Build history of the part. All positions in model axes, mm. A direction names the side the tool comes from. Give positions to 0.01 mm unless a question says otherwise; leave off trailing zeros. Write each loop counter-clockwise with the first axis right and the second up, starting at its lowest first coordinate (ties: lowest second). Pieces come first, ordered by that corner, then holes.
from build123d import *

# Parameters (mm, degrees)
SKETCH1_R                   = 25.4
BOSS_EXTRUDE1_DEPTH         = 152.4
SKETCH3_W                   = 25.4
SKETCH3_H                   = 88.9
CUT_EXTRUDE1_DEPTH          = 102.6
CUT_EXTRUDE1_DEPTH_BACK     = 102.6
F_1_4_0_25_DIAMETER_HOLE1_D = 6.35
SKETCH4_W                   = 25.4
SKETCH4_H                   = 101.6
CUT_EXTRUDE2_DEPTH          = 18.196861737


with BuildPart() as part:
    # Sketch1 → Boss-Extrude1 (new body)
    with BuildSketch(Plane.XY):
        with BuildLine():
            Line((-76.2, -38.1), (-76.2, -12.7))
            ThreePointArc((-76.2, -12.7), (-57.601280605, 32.201280605), (-12.7, 50.8))
            Line((-12.7, 50.8), (12.7, 50.8))
            ThreePointArc((12.7, 50.8), (57.601280605, 32.201280605), (76.2, -12.7))
            Line((76.2, -12.7), (76.2, -38.1))
            Line((76.2, -38.1), (101.6, -38.1))
            Line((101.6, -38.1), (101.6, -50.8))
            ThreePointArc((101.6, -50.8), (0, -55.296861637), (-101.6, -50.8))
            Line((-101.6, -50.8), (-101.6, -38.1))
            Line((-101.6, -38.1), (-76.2, -38.1))
        make_face()
        Circle(SKETCH1_R, mode=Mode.SUBTRACT)
    extrude(amount=BOSS_EXTRUDE1_DEPTH)

    # Sketch3 → Cut-Extrude1 (cut, two sides)
    with BuildSketch(Plane(origin=(0, 0, 0), x_dir=(0, 0, -1), z_dir=(1, 0, 0))) as cut_extrude1_sk:
        with Locations((-114.3, 6.35)):
            Rectangle(SKETCH3_W, SKETCH3_H)
        with Locations((-38.1, 6.35)):
            Rectangle(SKETCH3_W, SKETCH3_H)
    extrude(amount=CUT_EXTRUDE1_DEPTH, mode=Mode.SUBTRACT)
    extrude(cut_extrude1_sk.sketch, amount=-CUT_EXTRUDE1_DEPTH_BACK, mode=Mode.SUBTRACT)

    # 1/4 (0.25) Diameter Hole1 (through all)
    with Locations(Plane(origin=(0, -38.1, 0), x_dir=(1, 0, 0), z_dir=(0, 1, 0))):
        with Locations((-88.9, -12.7), (-88.9, -139.7), (88.9, -12.7), (88.9, -139.7)):
            Hole(F_1_4_0_25_DIAMETER_HOLE1_D / 2)

    # Sketch4 → Cut-Extrude2 (cut, through all)
    with BuildSketch(Plane(origin=(0, -38.1, 0), x_dir=(1, 0, 0), z_dir=(0, 1, 0))):
        with Locations((-88.9, -76.2)):
            Rectangle(SKETCH4_W, SKETCH4_H)
        with Locations((88.9, -76.2)):
            Rectangle(SKETCH4_W, SKETCH4_H)
    extrude(amount=-CUT_EXTRUDE2_DEPTH, mode=Mode.SUBTRACT)


solid = part.part
1. Drop flat-ended pins along their axis: pin 1 (20.5 mm diameter, centred on x = 94.5, z = 9.5, fed in from +Y); pin 2 (12.5 mm diameter, centred on y = -20, z = 146, fed in from -X); pin 3 (10 mm diameter, centred on y = 16.5, z = 70.5, fed in from -X). Give the stop position or say it passes through.
2. Mould opens along Z. For faces 5 (the face through (24, -13, 152.4)), 6 (the face through (-89, -45, 25.4)), 7 (the face through (76.2, -25, 13)) say: pulls with the +Z half, pulls with the -Z half, needs draft (parallel to the pull), parting line crosses it, or undercut.
3. Saw through at C-C on y = 0. Give the cut face in (x, z), plus the area to 3 significant figures.
4. 3-axis set-ups, long thin cutter, end or side, ignore diameter. For faces 1 (the face through (-89, -45, 127)), 2 (the face through (-76.2, -26, 13)), 3 (the face through (-1, -38.1, 38)), 4 (the face through (76.2, -25, 140)): which of +Z, -Z, +X, -X, +Y, -Y reach the whole face in a straight line?
5. Drill centre lines: line 1 along Z through (x, y) = (13, 29.5); line 2 along X through (y, z) = (-43.25, 139.7) (3 decimals); line 3 along Z through (x, y) = (-88.9, -41.5) (3 decimals). Where is each one in solid material? Low to high.
6. Saw through at D-D on z = 12.7. Give the cut face in (x, y) (3 decimals).
7. Saw through at B-B on x = 0. Give the cut face in (y, z), plus the area to 3 significant figures.
8. Saw through at A-A on z = 131. Give the cut face in (x, y), plus the area to 3 significant figures.
Outcome:
1. pin 1: stops at y = -38.1
1. pin 2: stops at x = -76.2
1. pin 3: stops at x = -71.41
2. face 5: pulls with the +Z half
2. face 6: undercut
2. face 7: needs draft
3. outline: (-74.92, 0) - (-25.4, 0) - (-25.4, 25.4) - (-74.92, 25.4) - close; (-74.92, 50.8) - (-25.4, 50.8) - (-25.4, 101.6) - (-74.92, 101.6) - close; (-74.92, 127) - (-25.4, 127) - (-25.4, 152.4) - (-74.92, 152.4) - close; (25.4, 0) - (74.92, 0) - (74.92, 25.4) - (25.4, 25.4) - close; (25.4, 50.8) - (74.92, 50.8) - (74.92, 101.6) - (25.4, 101.6) - close; (25.4, 127) - (74.92, 127) - (74.92, 152.4) - (25.4, 152.4) - close
3. area: 10,100 mm2
4. face 1: -X, +Y, -Y
4. face 2: +Z, -Z, -X, +Y
4. face 3: +X, -X, +Y
4. face 4: +Z, -Z, +X, +Y
5. line 1: z = 0 to 25.4, 50.8 to 101.6, 127 to 152.4
5. line 2: x = -101.6 to -92.075, -85.725 to 85.725, 92.075 to 101.6
5. line 3: z = 0 to 9.525, 15.875 to 25.4, 127 to 136.525, 142.875 to 152.4
6. outline: (-101.6, -50.8) arc R1150 ccw to (-92.075, -51.605) - (-92.075, -38.1) - (-101.6, -38.1) - close; (-85.725, -52.097) arc R1150 ccw to (85.725, -52.097) - (85.725, -38.1) - (76.2, -38.1) - (76.2, -12.7) arc R63.5 ccw to (12.7, 50.8) - (-12.7, 50.8) arc R63.5 ccw to (-76.2, -12.7) - (-76.2, -38.1) - (-85.725, -38.1) - close; (92.075, -51.605) arc R1150 ccw to (101.6, -50.8) - (101.6, -38.1) - (92.075, -38.1) - close; hole circle Ø50.8 at (0, 0)
7. outline: (-55.3, 0) - (-25.4, 0) - (-25.4, 25.4) - (-38.1, 25.4) - (-38.1, 50.8) - (-25.4, 50.8) - (-25.4, 101.6) - (-38.1, 101.6) - (-38.1, 127) - (-25.4, 127) - (-25.4, 152.4) - (-55.3, 152.4) - close; (25.4, 0) - (50.8, 0) - (50.8, 25.4) - (25.4, 25.4) - close; (25.4, 50.8) - (50.8, 50.8) - (50.8, 101.6) - (25.4, 101.6) - close; (25.4, 127) - (50.8, 127) - (50.8, 152.4) - (25.4, 152.4) - close
7. area: 6,490 mm2
8. outline: (-101.6, -50.8) arc R1150 ccw to (101.6, -50.8) - (101.6, -38.1) - (76.2, -38.1) - (76.2, -12.7) arc R63.5 ccw to (12.7, 50.8) - (-12.7, 50.8) arc R63.5 ccw to (-76.2, -12.7) - (-76.2, -38.1) - (-101.6, -38.1) - close; hole circle Ø50.8 at (0, 0)
8. area: 13,000 mm2
